Source: CAD feature listing. Evaluate the final solid. Frame: model axes, mm. A direction names the side the tool comes from. Give positions to 0.01 mm unless a question says otherwise; leave off trailing zeros. Loops run counter-clockwise (first coordinate to the right, second up) from the corner with the lowest first, then second, coordinate; pieces in that order, holes last. Notation, with made-up numbers: M 49.5,81.5 L 99.5,81.5 A18 cw 99.5,111.5 Z; hole C 68,12 d7. An arc over 180 degrees is marked long. Put each result on its own line as item: value.
from build123d import *

# Parameters (mm, degrees)
F1_DEPTH  = 63.5
F2_T      = -3.175
F4_DEPTH  = 9.525
F5_W      = 31.75
F5_H      = 15.875
F6_DEPTH  = 6.35
F8_DEPTH  = 60.325
F9_W      = 31.75
F9_H      = 28.575
F10_DEPTH = 9.525
F11_W     = 12.7
F11_H     = 22.225
F11_W_2   = 3.81
F11_H_2   = 15.875
F12_DEPTH = 25.654
F13_W     = 3.175
F13_H     = 22.225
F14_DEPTH = 127


with BuildPart() as f1:
    # F0 (on Top) → F1 (new body)
    with BuildSketch(Plane.XY):
        Polygon((107.95, 92.075), (-3.175, 92.075), (-107.95, -3.175), (-107.95, -92.075), (107.95, -92.075), align=None)
    extrude(amount=F1_DEPTH)

    # F2
    f2_openings = [f1.faces().sort_by_distance(p)[0] for p in [
        (10.480538, -8.657836, 0),
    ]]
    offset(amount=F2_T, openings=f2_openings)

    # F3 (on face) → F4 (join)
    with BuildSketch(Plane.XY.offset(63.5)):
        Polygon((107.95, 92.075), (-3.175, 92.075), (-107.95, -3.175), (-107.95, -92.075), (107.95, -92.075), align=None)
        Polygon((104.775, -88.9), (-104.775, -88.9), (-104.775, -4.579524), (-1.947523, 88.9), (104.775, 88.9), align=None, mode=Mode.SUBTRACT)
    extrude(amount=F4_DEPTH)

    # F5 (on face) → F6 (join)
    with BuildSketch(Plane.XY.offset(63.5)):
        with Locations((61.147683, 39.524323)):
            Rectangle(F5_W, F5_H)
        with Locations((61.147683, 0)):
            Rectangle(F5_W, F5_H)
        with Locations((61.147683, -39.524323)):
            Rectangle(F5_W, F5_H)
    extrude(amount=F6_DEPTH)

    # F7 (on face) → F8 (join, through all)
    with BuildSketch(Plane(origin=(0, 0, 60.325), x_dir=(1, 0, 0), z_dir=(0, 0, -1))):
        Polygon((104.775, 29.21), (104.775, 31.75), (40.541738, 31.75), (40.541738, 88.9), (38.001738, 88.9), (38.001738, 29.21), align=None)
    extrude(amount=F8_DEPTH)

    # F9 (on face) → F10 (join)
    with BuildSketch(Plane.YZ.offset(107.95)):
        with Locations((-47.625, 14.2875)):
            Rectangle(F9_W, F9_H)
    extrude(amount=F10_DEPTH)

    # F11 (on face) → F12 (cut)
    with BuildSketch(Plane.YZ.offset(117.475)):
        with Locations((-47.625, 13.6525)):
            Rectangle(F11_W, F11_H)
        with Locations((-58.7375, 14.5415)):
            Rectangle(F11_W_2, F11_H_2)
        with Locations((-36.5125, 14.5415)):
            Rectangle(F11_W_2, F11_H_2)
    extrude(amount=-F12_DEPTH, mode=Mode.SUBTRACT)

    # F13 (on face) → F14 (cut)
    with BuildSketch(Plane.XZ.offset(63.5)):
        with Locations((112.7125, 13.6525)):
            Rectangle(F13_W, F13_H)
    extrude(amount=-F14_DEPTH, mode=Mode.SUBTRACT)


solid = f1.part
1. Section query C-C (y = -26). Output: boundary loops of the cut face in (x, z) (3 decimals).
Found:
outline: M -107.95,0 L -104.775,0 L -104.775,60.325 L 104.775,60.325 L 104.775,0 L 107.95,0 L 107.95,73.025 L 104.775,73.025 L 104.775,63.5 L -104.775,63.5 L -104.775,73.025 L -107.95,73.025 Z
2. Material intervals for line 1 (Y direction, x = 101.5, z = 23) (3 decimals); line 2 (X direction, y = -53.5, z = 29) (3 decimals); line 3 (Y direction, x = 85, z = 70) (3 decimals), sorted ascending. Write a range as from..to.
Found:
line 1: -92.075..-88.9, -31.75..-29.21, 88.9..92.075
line 2: -107.95..-104.775, 38.002..40.542, 104.775..107.95
line 3: -92.075..-88.9, 88.9..92.075
3. Section query A-A (z = 66.5). State how many separate pieces and enclosed holes the cut face has, plus the area to 3 significant figures.
Found:
separate pieces: 4
enclosed holes: 1
area: 3,830 mm^2
4. Contact query for flat-ended pins moving along their axis: P1, Ø8, axis at x = 56.5, y = 3, coming from the +Z side; P2, Ø5, axis at y = 39, z = 67, coming from the -X side; P3, Ø6.5, axis at x = 111.5, y = -46, coming from the +Z side (3 decimals). Output: stop coordinate, or through.
Found:
P1: z = 69.85
P2: x = -64.31
P3: z = 28.575
5. Draft query along Z for faces 1 (the flat face through (114.3, -34, 13)), 2 (the flat face through (61, -39, 69.85)), 3 (the flat face through (38.002, -59, 31)). Return one class per face: pulls with the +Z half, pulls with the -Z half, needs draft (parallel to the pull), parting line crosses it, or undercut.
Found:
face 1: undercut
face 2: pulls with the +Z half
face 3: needs draft
6. Access query for faces 4 (the flat face through (-34, -88.9, 30)), 5 (the flat face through (108, -53.975, 13)), 6 (the flat face through (1, -88.9, 68)), 7 (the flat face through (111.125, -34, 13)). Directions: +Z, -Z, +X, -X, +Y, -Y. A direction counts if a zero-diameter tool reaches every point of the face in a straight line with its end or side. Return the directions, or none.
Found:
face 4: -Z
face 5: +X
face 6: +Z
face 7: +Y, -Y
7. Section query D-D (x = 98). Output: boundary loops of the cut face in (y, z) (3 decimals).
Found:
outline: M -92.075,0 L -88.9,0 L -88.9,60.325 L -31.75,60.325 L -31.75,0 L -29.21,0 L -29.21,60.325 L 88.9,60.325 L 88.9,0 L 92.075,0 L 92.075,73.025 L 88.9,73.025 L 88.9,63.5 L -88.9,63.5 L -88.9,73.025 L -92.075,73.025 Z
8. Section query B-B (z = 39). Output: boundary loops of the cut face in (x, y) (3 decimals).
Found:
outline: M -107.95,-92.075 L 107.95,-92.075 L 107.95,92.075 L -3.175,92.075 L -107.95,-3.175 Z; hole M -104.775,-88.9 L 38.002,-88.9 L 38.002,-29.21 L 104.775,-29.21 L 104.775,88.9 L -1.948,88.9 L -104.775,-4.58 Z; hole M 40.542,-88.9 L 104.775,-88.9 L 104.775,-31.75 L 40.542,-31.75 Z
